Geometry check sheet. Reference: drawing and pictorial views, mm from the part's lowest x, y, z. A direction names the side the tool comes from. Round coordinates to 2 decimals unless told otherwise and drop trailing zeros. Loops run counter-clockwise (first coordinate to the right, second up) from the corner with the lowest first, then second, coordinate; pieces in that order, holes last. Notation, with made-up numbers: (78, -3) - (95, -3) arc R6 cw to (95, 4) - close; hole circle Ø1 at (73.5, 32). An arc over 180 degrees is marked (long way). Answer as CSV lines item,"result". Start each with the question number.
1) Draft check along Z on the marked faces 1, 2, 3 and 4. Enter one of: released by +Z, released by -Z, zero draft, split by the parting line, or undercut.
2) Thickness scan on line 1 along Z through (x, y) = (6, 7); line 2 along Y through (x, z) = (20, 4.5); line 3 along Y through (x, z) = (20, 13.25). Record the ranges inside material, lowest first.
3) Cross-section at A-A on x = 20. Record the boundary of the cut face in (y, z).
4) Cross-section at D-D on x = 12.5. Record the boundary of the cut face in (y, z).
5) Cross-section at C-C on z = 17. Record the boundary of the cut face in (x, y).
6) Depth check by flat-ended pin: P1, Ø3, axis at y = 10.5, z = 9.5, coming from the +X side; P2, Ø9, axis at x = 18.5, y = 19, coming from the -Z side; P3, Ø1, axis at x = 33.5, z = 4, coming from the -Y side; P4, Ø2.5, axis at x = 20, y = 20, coming from the -Z side. Enter the tip coordinate at first touch or a pass-through.
7) Access from +Z, -Z, +X, -X, +Y, -Y to the whole of each face (thin tool, end or side, straight path). Record for the marked faces 5, 6 and 7.
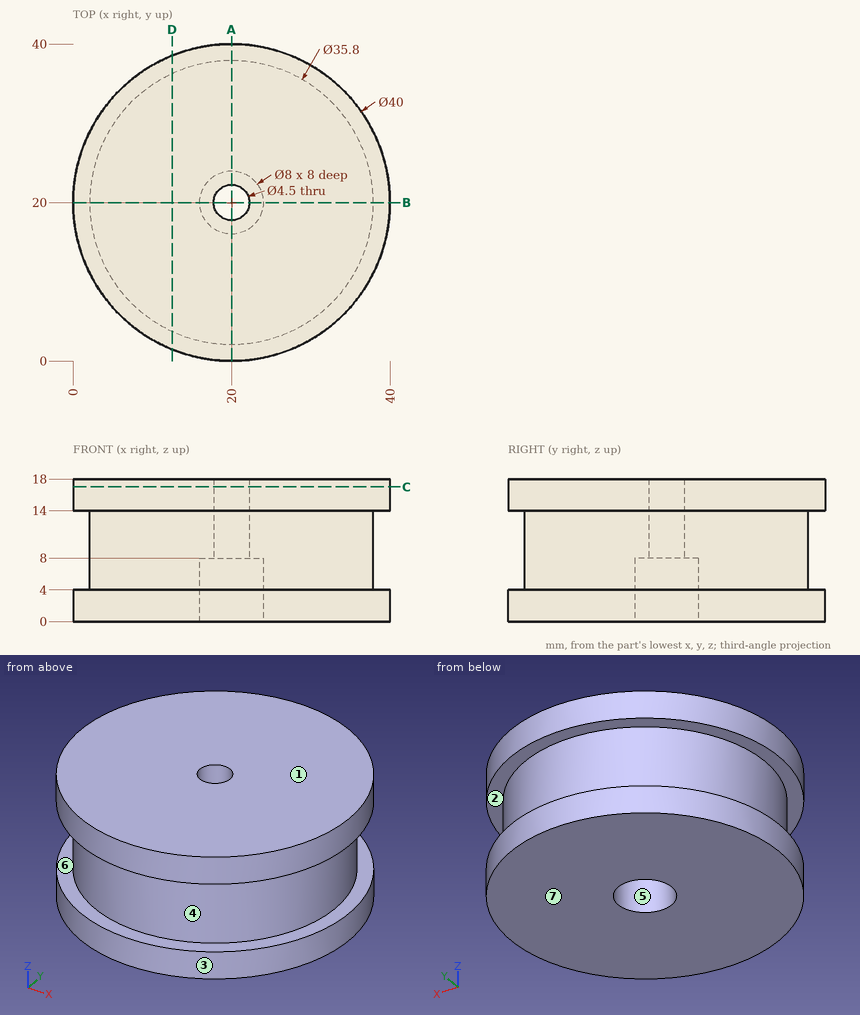
Answer block:
1,face 1,"released by +Z"
1,face 2,"undercut"
1,face 3,"zero draft"
1,face 4,"undercut"
2,line 1,"z = 0 to 4, 14 to 18"
2,line 2,"y = 2.1 to 16, 24 to 37.9"
2,line 3,"y = 2.1 to 17.75, 22.25 to 37.9"
3,outline,"(0, 0) - (16, 0) - (16, 8) - (17.75, 8) - (17.75, 18) - (0, 18) - (0, 14) - (2.1, 14) - (2.1, 4) - (0, 4) - close; (22.25, 8) - (24, 8) - (24, 0) - (40, 0) - (40, 4) - (37.9, 4) - (37.9, 14) - (40, 14) - (40, 18) - (22.25, 18) - close"
4,outline,"(1.46, 0) - (38.54, 0) - (38.54, 4) - (36.25, 4) - (36.25, 14) - (38.54, 14) - (38.54, 18) - (1.46, 18) - (1.46, 14) - (3.75, 14) - (3.75, 4) - (1.46, 4) - close"
5,outline,"circle Ø40 at (20, 20); hole circle Ø4.5 at (20, 20)"
6,P1,"stops at x = 36.01"
6,P2,"stops at z = 0"
6,P3,"stops at y = 4.8"
6,P4,"passes through"
7,face 5,"-Z"
7,face 6,"none"
7,face 7,"-Z, +X, -X, +Y, -Y"
